from build123d import *

# Parameters (mm, degrees)
F1_DEPTH = 1.5
F2_R     = 30
F3_R     = 0.5
F4_R     = 0.3


with BuildPart() as f1:
    # F0 (on Top) → F1 (new body)
    with BuildSketch(Plane.XY):
        Polygon((34.641016, 60), (-34.641016, 60), (-69.282032, 0), (-34.641016, -60), (34.641016, -60), (69.282032, 0), align=None)
        Polygon((0.65, -1.125833), (0.65, -51.125833), (-0.65, -51.125833), (-0.65, -1.125833), (-43.95127, -26.125833), (-44.60127, -25), (-1.3, 0), (-44.60127, 25), (-43.95127, 26.125833), (-0.65, 1.125833), (-0.65, 51.125833), (0.65, 51.125833), (0.65, 1.125833), (43.95127, 26.125833), (44.60127, 25), (1.3, 0), (44.60127, -25), (43.95127, -26.125833), align=None, mode=Mode.SUBTRACT)
    extrude(amount=F1_DEPTH)

    # F2
    f2_edges = [f1.edges().sort_by_distance(p)[0] for p in [
        (34.641016, 60, 0.75),
        (69.282032, 0, 0.75),
        (34.641016, -60, 0.75),
        (-34.641016, -60, 0.75),
        (-69.282032, 0, 0.75),
        (-34.641016, 60, 0.75),
    ]]
    fillet(f2_edges, radius=F2_R)

    # F3
    f3_edges = [f1.edges().sort_by_distance(p)[0] for p in [
        (43.95127, -26.125833, 0.75),
        (44.60127, -25, 0.75),
        (43.95127, 26.125833, 0.75),
        (44.60127, 25, 0.75),
        (-0.65, 51.125833, 0.75),
        (0.65, 51.125833, 0.75),
        (-44.60127, 25, 0.75),
        (-43.95127, 26.125833, 0.75),
        (-43.95127, -26.125833, 0.75),
        (-44.60127, -25, 0.75),
        (-0.65, -51.125833, 0.75),
        (0.65, -51.125833, 0.75),
    ]]
    fillet(f3_edges, radius=F3_R)

    # F4
    f4_edges = [f1.edges().sort_by_distance(p)[0] for p in [
        (-0.65, 1.125833, 0.75),
        (-1.3, 0, 0.75),
        (-0.65, -1.125833, 0.75),
        (0.65, 1.125833, 0.75),
        (1.3, 0, 0.75),
    ]]
    fillet(f4_edges, radius=F4_R)


solid = f1.part
Could you check a few things on this model? Use its own coordinates, in mm. A direction names the side the tool comes from. Give positions to 0.01 mm unless a question says otherwise; leave off trailing zeros. Order: outer loops, then holes, each group sorted by start corner. A loop starts at its lowest first (then second) coordinate and runs counter-clockwise, first axis right, second up. Notation, with made-up numbers: (26, 0.5) - (38, 0.5) arc R19 cw to (38, 7.5) - close; hole circle Ø8 at (-21, 5). An arc over 180 degrees is marked (long way). One line per item, written item: value. Start each with the question number.
1. Thinking about a two-plate mould opening in X: for faces 3 (the face through (64.64, 0.22, 0.76)), 4 (the face through (-32.51, -55.87, 0.76)), 5 (the face through (-22.01, -13.46, 0.74)), which applies, +X half, -X half, draft (parallel to the pull), parting line (faces both ways), or undercut?
2. If I drill on probe 1 along Y at (x, z) = (-9, 1.2); probe 2 along Y at (x, z) = (2, 0.2); probe 3 along X at (y, z) = (-16, 0.55), over which ranges is the centre line in solid material (lowest first)?
3. Imagine slicing it at B-B on y = -9. List the corners of the cut face in (x, z) for me.
4. For P1, Ø5, axis at x = -16, y = 46, coming from the -Z side, with a flat end and sliding along its axis, tell me the tip position at first contact or that it passes through.
5. Imagine slicing it at C-C on y = 43. List the corners of the cut face in (x, z) for me, plus the area to 3 significant figures.
6. For faces 1 (the face through (-52.083, -29.79, 0.74)), 2 (the face through (22.66, -12.33, 0.74)), which set-ups out of +Z, -Z, +X, -X, +Y, -Y let a thin tool reach every point of the face, with its end or its side?
7. Imagine slicing it at A-A on x = 34. List the corners of the cut face in (y, z) for me.
8. Imagine slicing it at D-D on y = 10. List the corners of the cut face in (x, z) for me, plus the area to 3 significant figures.
Values:
1. face 3: +X half
1. face 4: -X half
1. face 5: undercut
2. probe 1: -60 to -5.95, -4.45 to 4.45, 5.95 to 60
2. probe 2: -60 to -1.91, -0.4 to 0.4, 1.91 to 60
2. probe 3: -60.04 to -29.01, -26.41 to -0.65, 0.65 to 26.41, 29.01 to 60.04
3. outline: (-63.26, 0) - (-16.89, 0) - (-16.89, 1.5) - (-63.26, 1.5) - close; (-14.29, 0) - (-0.65, 0) - (-0.65, 1.5) - (-14.29, 1.5) - close; (0.65, 0) - (14.29, 0) - (14.29, 1.5) - (0.65, 1.5) - close; (16.89, 0) - (63.26, 0) - (63.26, 1.5) - (16.89, 1.5) - close
4. P1: z = 0
5. outline: (-44.46, 0) - (-0.65, 0) - (-0.65, 1.5) - (-44.46, 1.5) - close; (0.65, 0) - (44.46, 0) - (44.46, 1.5) - (0.65, 1.5) - close
5. area: 131 mm²
6. face 1: +Z, -Z, -X, -Y
6. face 2: +Z, -Z
7. outline: (-54.94, 0) - (-20.38, 0) - (-20.38, 1.5) - (-54.94, 1.5) - close; (-18.88, 0) - (18.88, 0) - (18.88, 1.5) - (-18.88, 1.5) - close; (20.38, 0) - (54.94, 0) - (54.94, 1.5) - (20.38, 1.5) - close
8. outline: (-62.93, 0) - (-18.62, 0) - (-18.62, 1.5) - (-62.93, 1.5) - close; (-16.02, 0) - (-0.65, 0) - (-0.65, 1.5) - (-16.02, 1.5) - close; (0.65, 0) - (16.02, 0) - (16.02, 1.5) - (0.65, 1.5) - close; (18.62, 0) - (62.93, 0) - (62.93, 1.5) - (18.62, 1.5) - close
8. area: 179 mm²
